Study the drawing (mm; zero at the part's minimum x, y, z) and answer. Give positions to 0.01 mm unless a question says otherwise; leave off trailing zeros. Write each loop counter-clockwise with the first axis right and the second up, starting at its lowest first coordinate (ties: lowest second). Pieces come first, ordered by that corner, then holes. Notation, with made-up numbers: (28, 39.25) -> (44, 39.25) arc R18 ccw to (44, 69.25) -> close; hole circle Ø8 at (-16, 51.25). An arc over 180 degrees is marked (long way). One line per question, with ' | ' between items.
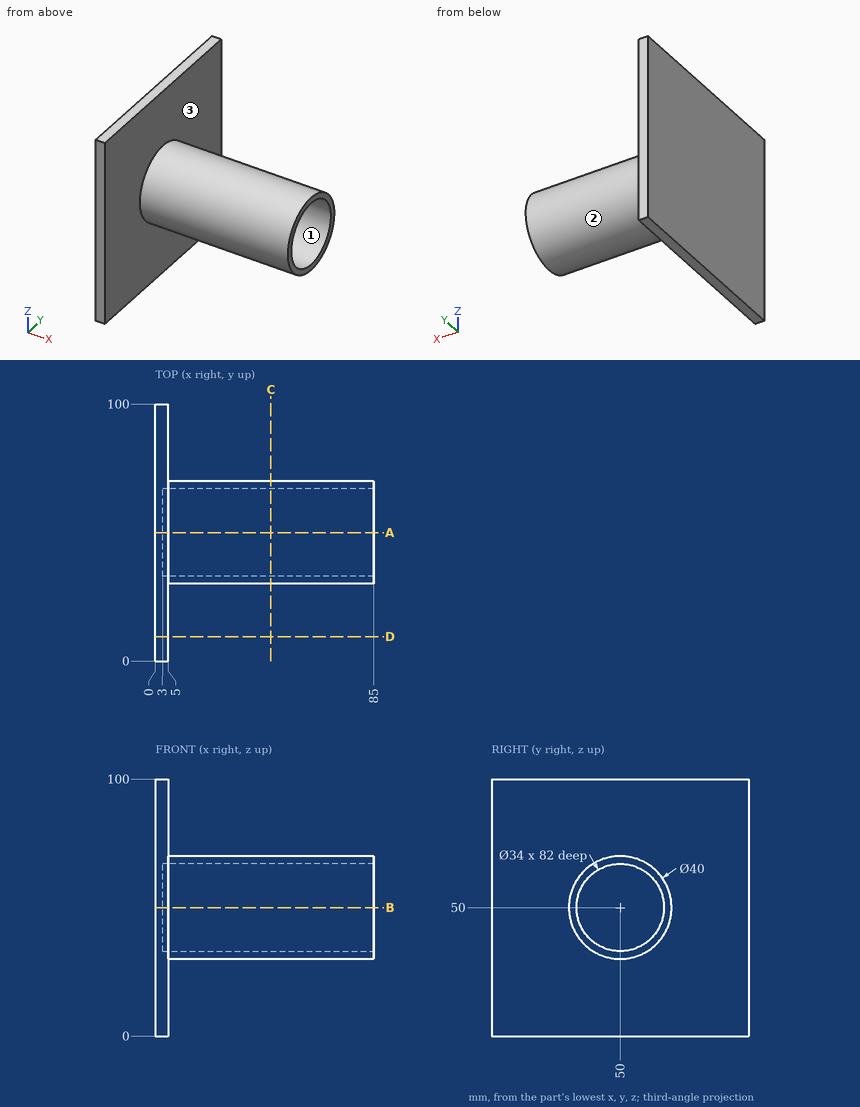
Item 1: Find section C-C (x = 45). Write down the section's boundary in (y, z).
Answers below:
outline: circle Ø40 at (50, 50); hole circle Ø34 at (50, 50)
Item 2: Consider line 1 (Y direction, x = 49.5, z = 51); line 2 (X direction, y = 81, z = 89). Determine where each line is inside the solid, lowest interval first. Write a range as [from, to].
Answers below:
line 1: [30.03, 33.03], [66.97, 69.97] | line 2: [0, 5]
Item 3: Find section D-D (y = 9.5). Write down the section's boundary in (x, z).
Answers below:
outline: (0, 0) -> (5, 0) -> (5, 100) -> (0, 100) -> close
Item 4: Flat-ended cylindrical pins translate along their axes: pin 1 (4 mm diameter, centred on y = 49, z = 60.5, fed in from -X); pin 2 (8 mm diameter, centred on x = 36.5, z = 32.5, fed in from +Y); pin 3 (5 mm diameter, centred on y = 31, z = 80, fed in from +X). Find the tip coordinate at first contact, or state that the pin passes through.
Answers below:
pin 1: x = 0 | pin 2: y = 64.76 | pin 3: x = 5
Item 5: Find section A-A (y = 50). Write down the section's boundary in (x, z).
Answers below:
outline: (0, 0) -> (5, 0) -> (5, 30) -> (85, 30) -> (85, 33) -> (3, 33) -> (3, 67) -> (85, 67) -> (85, 70) -> (5, 70) -> (5, 100) -> (0, 100) -> close
Item 6: Determine the mould class of the marked faces 1, 2 and 3 for opening direction Z: pulls with the +Z half, pulls with the -Z half, needs draft (parallel to the pull), parting line crosses it, or undercut.
Answers below:
face 1: undercut | face 2: parting line crosses it | face 3: needs draft
